Geometry check sheet. Reference: the model listing, model coordinates, mm. A direction names the side the tool comes from. Coordinates: 2 decimals unless noted, no trailing zeros. Order: outer loops, then holes, each group sorted by start corner. A loop starts at its lowest first (then second) coordinate and runs counter-clockwise, first axis right, second up.
```python
from build123d import *

# Parameters (mm, degrees)
F1_DEPTH = 24
F2_DEPTH = 15
F3_DEPTH = 12


with BuildPart() as f1:
    # F0 (on Front) → F1 (new body)
    with BuildSketch(Plane.XZ):
        Polygon((0, 36), (0, 0), (14, 20), (7.5, 36), align=None)
        Polygon((7.5, 36), (14, 20), (31, 20), (37.5, 36), align=None)
        Polygon((31, 20), (45, 0), (45, 36), (37.5, 36), align=None)
        Polygon((14, 20), (0, 0), (45, 0), (31, 20), align=None)
    extrude(amount=-F1_DEPTH)

    # F0 (on Front) → F2 (cut)
    with BuildSketch(Plane.XZ):
        Polygon((7.5, 36), (14, 20), (31, 20), (37.5, 36), align=None)
    extrude(amount=-F2_DEPTH, mode=Mode.SUBTRACT)

    # F0 (on Front) → F3 (join)
    with BuildSketch(Plane.XZ):
        Polygon((14, 20), (0, 0), (45, 0), (31, 20), align=None)
    extrude(amount=F3_DEPTH)


solid = f1.part
```
Item 1: Sectioned sample at B-B (z = 19). Record the cut outline in (x, y), and give its area (3 significant figures).
Item 2: Release check for a two-part mould opening along X. For faces 4 (the face through (5, 0, 22)), 5 (the face through (7, -6, 10)), 6 (the face through (23, 2, 20)) record: pulls with the +X half, pulls with the -X half, needs draft (parallel to the pull), parting line crosses it, or undercut.
Item 3: Depth check by flat-ended pin: P1, Ø4, axis at x = 26.5, z = 26.5, coming from the -Y side; P2, Ø8.5, axis at x = 26.5, y = 5, coming from the +Z side; P3, Ø1, axis at y = -1.5, z = 5, coming from the +X side. Enter the tip coordinate at first touch or a pass-through.
Item 4: Tool access check on faces 1 (the face through (34.204, 7.395, 27.888)), 2 (the face through (22, 24, 18)), 3 (the face through (39, 0, 22)). Record the directions out of +Z, -Z, +X, -X, +Y, -Y that give a thin tool (end or side, any length) a straight path to the whole face; none if there is none.
Item 5: Sectioned sample at D-D (y = -1.5). Record the cut outline in (x, z), and give its area (3 significant figures).
Item 6: Thickness scan on line 1 along Z through (x, y) = (14.5, 0.5); line 2 along Y through (x, z) = (3, 26); line 3 along X through (y, z) = (1.5, 25.5). Record the ranges inside material, lowest first.
Item 7: Sectioned sample at C-C (x = 17). Record the cut outline in (y, z), and give its area (3 significant figures).
Item 8: Sectioned sample at A-A (y = 6). Record the cut outline in (x, z).
Geometry check:
1. outline: (0, 0) - (13.3, 0) - (13.3, -12) - (31.7, -12) - (31.7, 0) - (45, 0) - (45, 24) - (0, 24) - close
1. area: 1,300 mm2
2. face 4: needs draft
2. face 5: pulls with the -X half
2. face 6: undercut
3. P1: stops at y = 15
3. P2: stops at z = 20
3. P3: stops at x = 41.85
4. face 1: +Z, -Y
4. face 2: +Z, -Z, +X, -X, +Y
4. face 3: +Z, +X, -Y
5. outline: (0, 0) - (45, 0) - (31, 20) - (14, 20) - close
5. area: 620 mm2
6. line 1: z = 0 to 20
6. line 2: y = 0 to 24
6. line 3: x = 0 to 11.77, 33.23 to 45
7. outline: (-12, 0) - (24, 0) - (24, 36) - (15, 36) - (15, 20) - (-12, 20) - close
7. area: 864 mm2
8. outline: (0, 0) - (45, 0) - (45, 36) - (37.5, 36) - (31, 20) - (14, 20) - (7.5, 36) - (0, 36) - close
